Source: CAD feature listing. Evaluate the final solid. Frame: model axes, mm. Give positions to 0.01 mm unless a question says otherwise; leave off trailing zeros. Write each loop counter-clockwise with the first axis right and the second up, starting at its lowest first coordinate (ties: lowest second). Pieces come first, ordered by that corner, then holes. Notation, with made-up numbers: (-8.75, 32.5) - (17.25, 32.5) arc R22 cw to (17.25, 42.5) - close; hole circle Ø11 at (63.5, -14). An arc over 180 degrees is marked (long way). Answer as a JSON object with one key per item and string values. Group by question number.
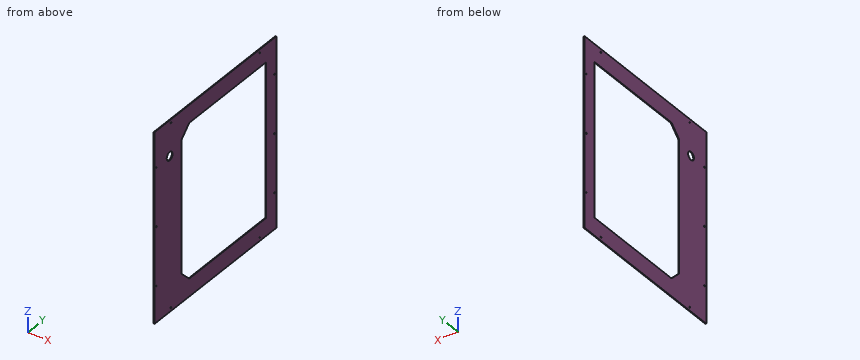
Autodesk Inventor part; units mm, degrees
ref_plane "YZ Plane" through (0, 0, 0) normal (1, 0, 0) x (0, 1, 0)
ref_plane "XZ Plane" through (0, 0, 0) normal (0, 1, 0) x (-1, 0, 0)
ref_plane "XY Plane" through (0, 0, 0) normal (0, 0, 1) x (1, 0, 0)
sketch "Sketch1" plane through (0, 0, 0) normal (1, 0, 0) x (0, 1, 0)
  line L0 (465, 411) -> (465, -123)
  line L1 (465, -123) -> (-15, -123)
  line L2 (-15, -123) -> (-15, 411)
  line L3 (-15, 411) -> (465, 411)
  circle A0 centre (400, -113.5) radius 1.75
  circle A1 centre (50, 401.5) radius 1.75
  circle A2 centre (400, 401.5) radius 1.75
  circle A3 centre (-7.5, -21) radius 1.75
  circle A4 centre (-7.5, 144) radius 1.75
  circle A5 centre (-7.5, 309) radius 1.75
  circle A6 centre (457.5, 144) radius 1.75
  circle A7 centre (457.5, -21) radius 1.75
  circle A8 centre (457.5, 309) radius 1.75
  circle A9 centre (50, -113.5) radius 1.75
  point P0 (0, 0)
extrude "Extrusion1" add sketch "Sketch1" along normal blind 2
sketch "Sketch2" plane through (0, 0, 0) normal (-1, 0, 0) x (0, 0, 1)
  line L0 (411, -15) -> (-123, -15)
  line L1 (411, 465) -> (411, -15)
  line L2 (-123, 465) -> (411, 465)
  line L3 (-123, -15) -> (-123, 465)
  circle A0 centre (-113.5, 50) radius 1.75
  circle A1 centre (-21, 457.5) radius 1.75
  circle A2 centre (144, 457.5) radius 1.75
  circle A3 centre (309, -7.5) radius 1.75
  circle A4 centre (144, -7.5) radius 1.75
  circle A5 centre (-21, -7.5) radius 1.75
  circle A6 centre (401.5, 400) radius 1.75
  circle A7 centre (401.5, 50) radius 1.75
  circle A8 centre (-113.5, 400) radius 1.75
  circle A9 centre (309, 457.5) radius 1.75
  line L4 (-73, 425) -> (361, 425)
  line L5 (361, 425) -> (361, 92)
  line L6 (361, 92) -> (-73, 92)
  line L7 (-73, 92) -> (-73, 425)
  point P0 (0, 0)
  dimension "d2" = 50
  dimension "d3" = 50
  dimension "d4" = 40
  dimension "d5" = 107
extrude "Extrusion2" cut sketch "Sketch2" against normal blind 2 contours L4 L5 L6 L7
chamfer "Chamfer1" distance 30 angle 45 2 edges at (1, 92, -73) (1, 92, 361)
sketch "Sketch3" plane through (0, 0, 0) normal (-1, 0, 0) x (0, 0, 1)
  line L0 (361, 425) -> (361, 122)
  line L1 (331, 92) -> (361, 122)
  line L2 (331, 92) -> (-43, 92)
  line L3 (-73, 122) -> (-43, 92)
  line L4 (-73, 122) -> (-73, 425)
  line L5 (-73, 425) -> (361, 425)
  line L6 (411, -15) -> (-123, -15)
  line L7 (411, 465) -> (411, -15)
  line L8 (-123, 465) -> (411, 465)
  line L9 (-123, -15) -> (-123, 465)
  circle A0 centre (-113.5, 50) radius 1.75
  circle A1 centre (-21, 457.5) radius 1.75
  circle A2 centre (144, 457.5) radius 1.75
  circle A3 centre (309, -7.5) radius 1.75
  circle A4 centre (144, -7.5) radius 1.75
  circle A5 centre (-21, -7.5) radius 1.75
  circle A6 centre (401.5, 400) radius 1.75
  circle A7 centre (401.5, 50) radius 1.75
  circle A8 centre (-113.5, 400) radius 1.75
  circle A9 centre (309, 457.5) radius 1.75
  circle A10 centre (311, 45) radius 11.5
  point P0 (0, 0)
  dimension "d11" = 23
  dimension "d12" = 60
  dimension "d13" = 100
extrude "Extrusion3" cut sketch "Sketch3" against normal through all contours A10
equation "\"d3\" = d2"
properties part number "Front Panel" material "Aluminum 6061"
Q1. Section A-A on z = 353. Return the cut outline in (x, y), then the cut area to 3 significant figures.
Q2. Ray query, probe 1 along Y at (x, z) = (1.4, 144); probe 2 along Z at (x, y) = (1.15, 457.5); probe 3 along Y at (x, z) = (1.15, -113.5). Return the intervals inside material, ascending. Write a range as [from, to].
Q3. Section C-C on x = 1.35. State how many separate pieces and enclosed holes the cut face has, then the cut area to 3 significant figures.
Q4. Section B-B on y = 341.5. Return the cut outline in (x, z), then the cut area to 3 significant figures.
Q5. First-contact query: pin 1 Ø5.5 at (y, z) = (-7.5, -21) entering from -X. Flat tip, straight axial feed; report the tip coordinate or a pass-through.
Taken from the geometry:
{
 "1": {"outline": "(0, -15) - (2, -15) - (2, 114) - (0, 114) - close; (0, 425) - (2, 425) - (2, 465) - (0, 465) - close", "area": "338 mm²"},
 "2": {"probe 1": "y = [-15, -9.25], [-5.75, 92], [425, 455.75], [459.25, 465]", "probe 2": "z = [-123, -22.75], [-19.25, 142.25], [145.75, 307.25], [310.75, 411]", "probe 3": "y = [-15, 48.25], [51.75, 398.25], [401.75, 465]"},
 "3": {"separate pieces": "1", "enclosed holes": "12", "area": "112,000 mm²"},
 "4": {"outline": "(0, -123) - (2, -123) - (2, -73) - (0, -73) - close; (0, 361) - (2, 361) - (2, 411) - (0, 411) - close", "area": "200 mm²"},
 "5": {"pin 1": "stops at x = 0"}
}
